Verification items for the finished model (mm, model axes). A direction names the side the tool comes from. Round coordinates to 2 decimals unless told otherwise and drop trailing zeros. Loops run counter-clockwise (first coordinate to the right, second up) from the corner with the lowest first, then second, coordinate; pieces in that order, holes last. Notation, with made-up numbers: (20, 13.5) - (35, 13.5) arc R11 cw to (35, 34.5) - close; hole circle Ø4 at (28.5, 49.25). An arc over 180 degrees is marked (long way). Use a Markdown table: item, result. Add a question column.
Autodesk Inventor part; units mm, degrees
ref_plane "YZ Plane" through (0, 0, 0) normal (1, 0, 0) x (0, 1, 0)
ref_plane "XZ Plane" through (0, 0, 0) normal (0, 1, 0) x (-1, 0, 0)
ref_plane "XY Plane" through (0, 0, 0) normal (0, 0, 1) x (1, 0, 0)
sketch "Boceto1" plane through (0, 0, 0) normal (0, 0, 1) x (1, 0, 0)
  line L0 (-18, -12) -> (18, -12)
  line L1 (18, -12) -> (18, 12)
  line L2 (18, 12) -> (-18, 12)
  line L3 (-18, 12) -> (-18, -12)
  line L4 (-18, -12) -> (18, 12) construction
  line L5 (18, -12) -> (-18, 12) construction
  circle A0 centre (0, 0) radius 9.525
  line L6 (-15, -9) -> (15, -9)
  line L7 (15, -9) -> (15, 9)
  line L8 (15, 9) -> (-15, 9)
  line L9 (-15, 9) -> (-15, -9)
  line L10 (-15, -9) -> (15, 9) construction
  line L11 (15, -9) -> (-15, 9) construction
  dimension "d0" = 36
  dimension "d1" = 24
  dimension "d2" = 19.05
  dimension "d3" = 30
  dimension "d4" = 18
extrude "Extrusión1" add sketch "Boceto1" along normal blind 4 contours L3 L2 L1 L0 | A0 L6 L8 | A0 L8 L7 L6 | L8 A0 | A0 L6 | A0 L6 L9 L8
sketch "Boceto2" plane through (0, 0, 4) normal (0, 0, 1) x (1, 0, 0)
  circle A0 centre (0, 0) radius 9.525
  dimension "d7" = 19.05
extrude "Extrusión2" add sketch "Boceto2" along normal blind 18
sketch "Boceto3" plane through (0, 0, 22) normal (0, 0, 1) x (1, 0, 0)
  point P0 (0, 0)
  point P1 (0, 0)
hole "Agujero1" at (0, 0, 22) direction (0, 0, -1) diameter 12 depth 8
sketch "Boceto4" plane through (0, 0, 0) normal (0, 0, -1) x (-1, 0, 0)
  line L0 (15, -9) -> (-15, -9)
  line L1 (-15, -9) -> (-15, 9)
  line L2 (-15, 9) -> (15, 9)
  line L3 (15, 9) -> (15, -9)
  line L4 (15, -9) -> (-15, 9) construction
  line L5 (-15, -9) -> (15, 9) construction
  point P0 (0, 0)
  dimension "d17" = 30
  dimension "d18" = 18
hole "Agujero2" at (15, 9, 0) at (15, -9, 0) at (-15, 9, 0) at (-15, -9, 0) direction (0, 0, 1) diameter 3 depth 8 tip angle 118
properties part number "SoporteVarillaZ"
Q1. Set-up check for faces 5 (the face through (0, 0, 14)), 6 (the face through (-0.1, -6.2, 22)): record each of +Z, -Z, +X, -X, +Y, -Y from which the full face is reachable in a straight line by a thin tool's end or side.
Q2. Thickness scan on line 1 along X through (y, z) = (-9, 1.6); line 2 along Y through (x, z) = (15, 2.15); line 3 along Y through (x, z) = (0, 16.5) (3 decimals). Record the ranges inside material, lowest first.
Q3. Release check for a two-part mould opening along X. For faces 1 (the face through (-7.559, 5.796, 12.874)), 2 (the face through (-18, 0, 2)), 3 (the face through (0, -12, 2)), 4 (the face through (-15.07, -10.5, 2.03)) record: +X half, -X half, draft (parallel to the pull), parting line (faces both ways), or undercut.
Q4. Section check B-B on y = -9. Record the cut outline in (x, z), plus the area to 3 significant figures.
Q5. Section check C-C on y = 0. Record the cut outline in (x, z) (3 decimals).
Q6. Go/stop test with flat-tipped pins: pin 1 Ø12 at (x, z) = (-8.5, 18) entering from -Y; pin 2 Ø1.8 at (x, y) = (15, 9) entering from +Z; pin 3 Ø1 at (x, z) = (0, 11) entering from +Y (3 decimals); pin 4 Ø3 at (y, z) = (-7.5, 8) entering from -X. Record where each tip stops, or that it passes through.
Q7. Section check A-A on x = -15. Record the cut outline in (y, z), plus the area to 3 significant figures.
Q8. Section check D-D on x = 0. Record the cut outline in (y, z) (3 decimals), plus the area to 3 significant figures.
Determined:
| question | item | result |
|---|---|---|
| 1 | face 5 | +Z |
| 1 | face 6 | +Z, +X, -X, +Y, -Y |
| 2 | line 1 | x = -18 to -16.5, -13.5 to 13.5, 16.5 to 18 |
| 2 | line 2 | y = -12 to -10.5, -7.5 to 7.5, 10.5 to 12 |
| 2 | line 3 | y = -9.525 to -6, 6 to 9.525 |
| 3 | face 1 | parting line |
| 3 | face 2 | -X half |
| 3 | face 3 | draft |
| 3 | face 4 | undercut |
| 4 | outline | (-18, 0) - (-16.5, 0) - (-16.5, 4) - (-18, 4) - close; (-13.5, 0) - (13.5, 0) - (13.5, 4) - (3.12, 4) - (3.12, 22) - (-3.12, 22) - (-3.12, 4) - (-13.5, 4) - close; (16.5, 0) - (18, 0) - (18, 4) - (16.5, 4) - close |
| 4 | area | 232 mm² |
| 5 | outline | (-18, 0) - (18, 0) - (18, 4) - (9.525, 4) - (9.525, 22) - (6, 22) - (6, 14) - (-6, 14) - (-6, 22) - (-9.525, 22) - (-9.525, 4) - (-18, 4) - close |
| 6 | pin 1 | stops at y = -9.19 |
| 6 | pin 2 | passes through |
| 6 | pin 3 | stops at y = 9.525 |
| 6 | pin 4 | stops at x = -7.4 |
| 7 | outline | (-12, 0) - (-10.5, 0) - (-10.5, 4) - (-12, 4) - close; (-7.5, 0) - (7.5, 0) - (7.5, 4) - (-7.5, 4) - close; (10.5, 0) - (12, 0) - (12, 4) - (10.5, 4) - close |
| 7 | area | 72.0 mm² |
| 8 | outline | (-12, 0) - (12, 0) - (12, 4) - (9.525, 4) - (9.525, 22) - (6, 22) - (6, 14) - (-6, 14) - (-6, 22) - (-9.525, 22) - (-9.525, 4) - (-12, 4) - close |
| 8 | area | 343 mm² |
